Build history of the part. All positions in model axes, mm. A direction names the side the tool comes from. Round coordinates to 2 decimals unless told otherwise and drop trailing zeros. Order: outer loops, then holes, each group sorted by start corner. A loop starts at its lowest first (then second) coordinate and runs counter-clockwise, first axis right, second up. Notation, with made-up numbers: (12.5, 47.5) -> (31.5, 47.5) arc R17 ccw to (31.5, 77.5) -> close; hole circle Ø7 at (38.5, -22.75). An arc over 180 degrees is marked (long way). Answer as a JSON object with one key per item and string values.
from build123d import *

# Parameters (mm, degrees)
SKETCH1_R           = 34
SKETCH1_R_2         = 26.1
BOSS_EXTRUDE1_DEPTH = 0.5
SKETCH2_R           = 35.5
SKETCH2_R_2         = 26.1
BOSS_EXTRUDE2_DEPTH = 2
SKETCH3_R           = 38.5
SKETCH3_R_2         = 25
BOSS_EXTRUDE3_DEPTH = 2.5
CHAMFER1_SIZE       = 0.5
SKETCH4_R           = 1.65
SKETCH4_R_2         = 2.5
CUT_EXTRUDE1_DEPTH  = 55.676320286
SKETCH6_R           = 3.65
SKETCH6_R_2         = 1.65
CUT_EXTRUDE2_DEPTH  = 3
BOSS_EXTRUDE4_START = 2
SKETCH7_R           = 4.5
SKETCH7_R_2         = 2.5
BOSS_EXTRUDE4_DEPTH = 2


with BuildPart() as part:
    # Sketch1 → Boss-Extrude1 (new body)
    with BuildSketch(Plane(origin=(0, 0, 0), x_dir=(1, 0, 0), z_dir=(0, 1, 0))):
        with Locations(Location((0, 0, 0), (0, 0, 270))):
            Circle(SKETCH1_R)
        with Locations(Location((0, 0, 0), (0, 0, 270))):
            Circle(SKETCH1_R_2, mode=Mode.SUBTRACT)
    extrude(amount=BOSS_EXTRUDE1_DEPTH)

    # Sketch2 → Boss-Extrude2 (add)
    with BuildSketch(Plane(origin=(0, 0.5, 0), x_dir=(1, 0, 0), z_dir=(0, 1, 0))):
        with Locations(Location((0, 0, 0), (0, 0, 270))):
            Circle(SKETCH2_R)
        with Locations(Location((0, 0, 0), (0, 0, 270))):
            Circle(SKETCH2_R_2, mode=Mode.SUBTRACT)
    extrude(amount=BOSS_EXTRUDE2_DEPTH)

    # Sketch3 → Boss-Extrude3 (add)
    with BuildSketch(Plane(origin=(0, 2.5, 0), x_dir=(1, 0, 0), z_dir=(0, 1, 0))):
        with Locations(Location((0, 0, 0), (0, 0, 270))):
            Circle(SKETCH3_R)
        with Locations(Location((0, 0, 0), (0, 0, 270))):
            Circle(SKETCH3_R_2, mode=Mode.SUBTRACT)
    extrude(amount=BOSS_EXTRUDE3_DEPTH)

    # Chamfer1
    chamfer1_edges = [part.edges().sort_by_distance(p)[0] for p in [
        (0, 0.5, -34),
    ]]
    chamfer(chamfer1_edges, length=CHAMFER1_SIZE - 0.0001)  # a hair under: the kernel refuses the full size

    # Sketch4 → Cut-Extrude1 (cut, through all)
    with BuildSketch(Plane(origin=(0, 5, 0), x_dir=(1, 0, 0), z_dir=(0, 1, 0))):
        with Locations(Location((0, 30, 0), (0, 0, 270))):
            Circle(SKETCH4_R)
        with Locations(Location((21.213203436, 21.213203436, 0), (0, 0, 270))):
            Circle(SKETCH4_R_2)
        with Locations(Location((30, 0, 0), (0, 0, 270))):
            Circle(SKETCH4_R)
        with Locations(Location((21.213203436, -21.213203436, 0), (0, 0, 270))):
            Circle(SKETCH4_R_2)
        with Locations(Location((0, -30, 0), (0, 0, 270))):
            Circle(SKETCH4_R)
        with Locations(Location((-21.213203436, -21.213203436, 0), (0, 0, 270))):
            Circle(SKETCH4_R_2)
        with Locations(Location((-30, 0, 0), (0, 0, 270))):
            Circle(SKETCH4_R)
        with Locations(Location((-21.213203436, 21.213203436, 0), (0, 0, 270))):
            Circle(SKETCH4_R_2)
    extrude(amount=-CUT_EXTRUDE1_DEPTH, mode=Mode.SUBTRACT)

    # Sketch6 → Cut-Extrude2 (cut)
    # profile 1 of 4: a face of its own
    with BuildSketch(Plane(origin=(0, 5, 0), x_dir=(1, 0, 0), z_dir=(0, 1, 0))):
        with Locations(Location((0, -30, 0), (0, 0, 270))):
            Circle(SKETCH6_R)
        with Locations(Location((0, -30, 0), (0, 0, 270))):
            Circle(SKETCH6_R_2, mode=Mode.SUBTRACT)
    # profile 2 of 4: a face of its own
    with BuildSketch(Plane(origin=(0, 5, 0), x_dir=(1, 0, 0), z_dir=(0, 1, 0))):
        with Locations(Location((30, 0, 0), (0, 0, 270))):
            Circle(SKETCH6_R)
        with Locations(Location((30, 0, 0), (0, 0, 270))):
            Circle(SKETCH6_R_2, mode=Mode.SUBTRACT)
    # profile 3 of 4: a face of its own
    with BuildSketch(Plane(origin=(0, 5, 0), x_dir=(1, 0, 0), z_dir=(0, 1, 0))):
        with Locations(Location((0, 30, 0), (0, 0, 270))):
            Circle(SKETCH6_R)
        with Locations(Location((0, 30, 0), (0, 0, 270))):
            Circle(SKETCH6_R_2, mode=Mode.SUBTRACT)
    # profile 4 of 4: a face of its own
    with BuildSketch(Plane(origin=(0, 5, 0), x_dir=(1, 0, 0), z_dir=(0, 1, 0))):
        with Locations(Location((-30, 0, 0), (0, 0, 270))):
            Circle(SKETCH6_R)
        with Locations(Location((-30, 0, 0), (0, 0, 270))):
            Circle(SKETCH6_R_2, mode=Mode.SUBTRACT)
    extrude(amount=-CUT_EXTRUDE2_DEPTH, mode=Mode.SUBTRACT)

    # Sketch7 → Boss-Extrude4 (add)
    # profile 1 of 4: a face of its own
    with BuildSketch(Plane(origin=(0, 5, 0), x_dir=(1, 0, 0), z_dir=(0, 1, 0)).offset(BOSS_EXTRUDE4_START)):
        with Locations(Location((-21.213203436, 21.213203436, 0), (0, 0, 270))):
            Circle(SKETCH7_R)
        with Locations(Location((-21.213203436, 21.213203436, 0), (0, 0, 270))):
            Circle(SKETCH7_R_2, mode=Mode.SUBTRACT)
    # profile 2 of 4: a face of its own
    with BuildSketch(Plane(origin=(0, 5, 0), x_dir=(1, 0, 0), z_dir=(0, 1, 0)).offset(BOSS_EXTRUDE4_START)):
        with Locations(Location((21.213203436, 21.213203436, 0), (0, 0, 270))):
            Circle(SKETCH7_R)
        with Locations(Location((21.213203436, 21.213203436, 0), (0, 0, 270))):
            Circle(SKETCH7_R_2, mode=Mode.SUBTRACT)
    # profile 3 of 4: a face of its own
    with BuildSketch(Plane(origin=(0, 5, 0), x_dir=(1, 0, 0), z_dir=(0, 1, 0)).offset(BOSS_EXTRUDE4_START)):
        with Locations(Location((21.213203436, -21.213203436, 0), (0, 0, 270))):
            Circle(SKETCH7_R)
        with Locations(Location((21.213203436, -21.213203436, 0), (0, 0, 270))):
            Circle(SKETCH7_R_2, mode=Mode.SUBTRACT)
    # profile 4 of 4: a face of its own
    with BuildSketch(Plane(origin=(0, 5, 0), x_dir=(1, 0, 0), z_dir=(0, 1, 0)).offset(BOSS_EXTRUDE4_START)):
        with Locations(Location((-21.213203436, -21.213203436, 0), (0, 0, 270))):
            Circle(SKETCH7_R)
        with Locations(Location((-21.213203436, -21.213203436, 0), (0, 0, 270))):
            Circle(SKETCH7_R_2, mode=Mode.SUBTRACT)
    extrude(amount=-BOSS_EXTRUDE4_DEPTH)


solid = part.part
1) Which spindle directions (+Z, -Z, +X, -X, +Y, -Y) get a long thin tool onto all of the face, cutting with end or side? Do faces 1 (the face through (0.16, 3.521, 26.354)), 2 (the face through (7.509, 3.732, 23.846)). Say none if no direction does.
Checked values:
{"face 1": "+Y", "face 2": "+Y, -Y"}
2) Pull direction Z, two halves, no side cores. Call faces 3 (the face through (21.32, 3.55, -23.71)), 4 (the face through (19, 7, 23)): pulls with the +Z half, pulls with the -Z half, needs draft (parallel to the pull), parting line crosses it, or undercut.
Checked values:
{"face 3": "undercut", "face 4": "needs draft"}
3) Cut at B-B, the plane z = 0. Count the separate pieces of the cut face and the enclosed holes in it, plus the area to 4 significant figures.
Checked values:
{"separate pieces": "4", "enclosed holes": "0", "area": "56.25 mm²"}
4) Probe L1, parallel to Z at x = 20.5, y = 6.25; L2, parallel to Z at x = 19, y = 5.75; L3, parallel to Y at x = 9.5, z = -30.5. List the from-to ranges inside material, lowest first. Write a range as from..to.
Checked values:
{"L1": "z = -25.66..-23.61, -18.82..-16.77, 16.77..18.82, 23.61..25.66", "L2": "z = -25.13..-22.38, -20.05..-17.3, 17.3..20.05, 22.38..25.13", "L3": "y = 0..5"}
5) Flat gauge pins, fed straight in: pin 1 Ø6 at (x, z) = (-0.5, -28.5) entering from +Y; pin 2 Ø4 at (x, z) = (30, 0) entering from +Y; pin 3 Ø1.5 at (y, z) = (3.5, -6.5) entering from +X. Where does each tip first touch, or does it go through?
Checked values:
{"pin 1": "stops at y = 5", "pin 2": "stops at y = 2", "pin 3": "stops at x = 38.07"}
6) Cut at A-A, the plane y = 6. Give the cut face in (x, z), plus the area to 3 significant figures.
Checked values:
{"outline": "circle Ø9 at (-21.21, -21.21); circle Ø9 at (-21.21, 21.21); circle Ø9 at (21.21, -21.21); circle Ø9 at (21.21, 21.21); hole circle Ø5 at (-21.21, -21.21); hole circle Ø5 at (-21.21, 21.21); hole circle Ø5 at (21.21, -21.21); hole circle Ø5 at (21.21, 21.21)", "area": "176 mm²"}
